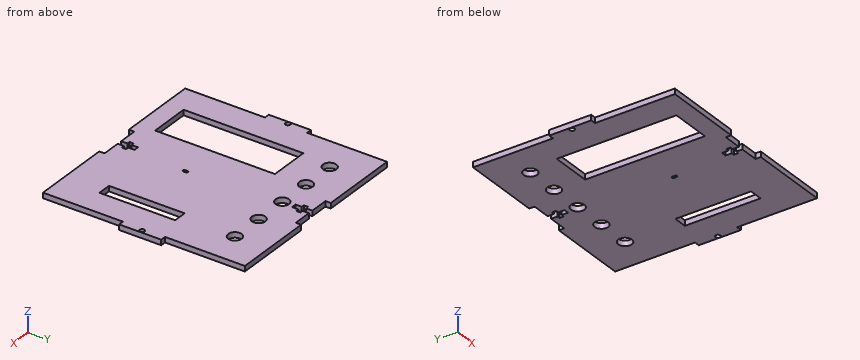
from build123d import *

# Parameters (mm, degrees)
SKETCH1_R           = 1.47
BOSS_EXTRUDE1_DEPTH = 1.5875
SKETCH3_W           = 8
SKETCH3_H           = 45
CUT_EXTRUDE1_DEPTH  = 88.184638842
SKETCH4_W           = 24
SKETCH4_H           = 71.2
CUT_EXTRUDE2_DEPTH  = 88.184638842
CUT_EXTRUDE4_DEPTH  = 88.184638842
SKETCH6_R           = 4
CUT_EXTRUDE5_DEPTH  = 88.184638842


with BuildPart() as part:
    # Sketch1 → Boss-Extrude1 (new, symmetric)
    with BuildSketch(Plane.XY):
        Polygon((-12.5, 60), (-60, 60), (-60, 12.5), (-63.175, 12.5), (-63.175, -12.5), (-60, -12.5), (-60, -60), (-12.5, -60), (-12.5, -56.825), (-1.47, -56.825), (-1.47, -53.125), (-3.25, -53.125), (-3.25, -50.525), (-1.47, -50.525), (-1.47, -46.825), (1.47, -46.825), (1.47, -50.525), (3.25, -50.525), (3.25, -53.125), (1.47, -53.125), (1.47, -56.825), (12.5, -56.825), (12.5, -60), (60, -60), (60, -12.5), (63.175, -12.5), (63.175, 12.5), (60, 12.5), (60, 60), (12.5, 60), (12.5, 56.825), (1.47, 56.825), (1.47, 53.125), (3.25, 53.125), (3.25, 50.525), (1.47, 50.525), (1.47, 46.825), (-1.47, 46.825), (-1.47, 50.525), (-3.25, 50.525), (-3.25, 53.125), (-1.47, 53.125), (-1.47, 56.825), (-12.5, 56.825), align=None)
        with Locations((-61.5875, 0)):
            Circle(SKETCH1_R, mode=Mode.SUBTRACT)
        with Locations(Location((61.5875, 0, 0), (0, 0, 180))):
            Circle(SKETCH1_R, mode=Mode.SUBTRACT)
    extrude(amount=BOSS_EXTRUDE1_DEPTH, both=True)

    # Sketch3 → Cut-Extrude1 (cut, through all)
    with BuildSketch(Plane(origin=(0, 0, -1.5875), x_dir=(-1, 0, 0), z_dir=(0, 0, -1))):
        with Locations((-40.3, -15)):
            Rectangle(SKETCH3_W, SKETCH3_H)
    extrude(amount=-CUT_EXTRUDE1_DEPTH, mode=Mode.SUBTRACT)

    # Sketch4 → Cut-Extrude2 (cut, through all)
    with BuildSketch(Plane(origin=(0, 0, -1.5875), x_dir=(-1, 0, 0), z_dir=(0, 0, -1))):
        with Locations((31.2, -13.494459363)):
            Rectangle(SKETCH4_W, SKETCH4_H)
    extrude(amount=-CUT_EXTRUDE2_DEPTH, mode=Mode.SUBTRACT)

    # Sketch5 → Cut-Extrude4 (cut, through all)
    with BuildSketch(Plane(origin=(0, 0, -1.5875), x_dir=(-1, 0, 0), z_dir=(0, 0, -1))):
        with BuildLine():
            Line((-3.324117887, -16.45), (-3.949848491, -16.45))
            ThreePointArc((-3.949848491, -16.45), (-4.214195834, -16.350200736), (-4.346634826, -16.10060241))
            ThreePointArc((-4.346634826, -16.10060241), (-4.416532026, -15), (-4.346634826, -13.89939759))
            ThreePointArc((-4.346634826, -13.89939759), (-4.214195834, -13.649799264), (-3.949848491, -13.55))
            Line((-3.949848491, -13.55), (-3.324117887, -13.55))
            ThreePointArc((-3.324117887, -13.55), (-3.041275174, -13.667157288), (-2.924117887, -13.95))
            Line((-2.924117887, -13.95), (-2.924117887, -16.05))
            ThreePointArc((-2.924117887, -16.05), (-3.041275174, -16.332842712), (-3.324117887, -16.45))
        make_face()
    extrude(amount=-CUT_EXTRUDE4_DEPTH, mode=Mode.SUBTRACT)

    # Sketch6 → Cut-Extrude5 (cut, through all)
    with BuildSketch(Plane(origin=(0, 0, -1.5875), x_dir=(-1, 0, 0), z_dir=(0, 0, -1))):
        with Locations((40, 40)):
            Circle(SKETCH6_R)
        with Locations((20, 40)):
            Circle(SKETCH6_R)
        with Locations((0, 40)):
            Circle(SKETCH6_R)
        with Locations((-20, 40)):
            Circle(SKETCH6_R)
        with Locations((-40, 40)):
            Circle(SKETCH6_R)
    extrude(amount=-CUT_EXTRUDE5_DEPTH, mode=Mode.SUBTRACT)


solid = part.part
CAD build for the part. Positions are in the model's coordinates, mm. Round coordinates to 2 decimals unless told otherwise and drop trailing zeros. Order: outer loops, then holes, each group sorted by start corner. A loop starts at its lowest first (then second) coordinate and runs counter-clockwise, first axis right, second up. Notation, with made-up numbers: (-26, 62) -> (23, 62) arc R22 cw to (23, 81) -> close; hole circle Ø4 at (-2.5, -22). An arc over 180 degrees is marked (long way). Write item = value, one per line. Start each with the question number.
(1) Cut at A-A, the plane y = -39. List the corners of the cut face in (x, z).
(2) Cut at B-B, the plane x = 0. List the corners of the cut face in (y, z) (1 decimal), then the cut area to 3 significant figures.
(3) Pin check, flat tips, straight feed: P1, Ø0.9, axis at x = 2, z = 0.5, coming from the +Y side (3 decimals); P2, Ø1.6, axis at y = -48.5, z = 0.5, coming from the +X side; P3, Ø1.5, axis at y = -23.5, z = 1, coming from the -X side; P4, Ø1.5, axis at x = 43.5, y = -3, coming from the +Z side. Stop position of each tip, or through.
(4) Cut at D-D, the plane x = -40. List the corners of the cut face in (y, z).
(5) Probe line 1 (Y direction, x = -20.5, z = -0.7); line 2 (X direction, y = -7, z = 0.3) (3 decimals); line 3 (X direction, y = -31.5, z = 0.7). List the from-to ranges inside material, lowest first. Write a range as [from, to].
(6) Cut at C-C, the plane y = 40. List the corners of the cut face in (x, z).
Model answer:
q1.outline = (-60, -1.59) -> (-43.2, -1.59) -> (-43.2, 1.59) -> (-60, 1.59) -> close; (-19.2, -1.59) -> (60, -1.59) -> (60, 1.59) -> (-19.2, 1.59) -> close
q2.outline = (-46.8, -1.6) -> (36, -1.6) -> (36, 1.6) -> (-46.8, 1.6) -> close; (44, -1.6) -> (46.8, -1.6) -> (46.8, 1.6) -> (44, 1.6) -> close
q2.area = 272 mm2
q3.P1 = 56.825
q3.P2 = 60
q3.P3 = -60
q3.P4 = through
q4.outline = (-60, -1.59) -> (-49.09, -1.59) -> (-49.09, 1.59) -> (-60, 1.59) -> close; (22.11, -1.59) -> (36, -1.59) -> (36, 1.59) -> (22.11, 1.59) -> close; (44, -1.59) -> (60, -1.59) -> (60, 1.59) -> (44, 1.59) -> close
q5.line_1 = [-60, -49.09], [22.11, 36.03], [43.97, 60]
q5.line_2 = [-63.175, -43.2], [-19.2, 36.3], [44.3, 63.175]
q5.line_3 = [-60, -43.2], [-19.2, 36.3], [44.3, 60]
q6.outline = (-60, -1.59) -> (-44, -1.59) -> (-44, 1.59) -> (-60, 1.59) -> close; (-36, -1.59) -> (-24, -1.59) -> (-24, 1.59) -> (-36, 1.59) -> close; (-16, -1.59) -> (-4, -1.59) -> (-4, 1.59) -> (-16, 1.59) -> close; (4, -1.59) -> (16, -1.59) -> (16, 1.59) -> (4, 1.59) -> close; (24, -1.59) -> (36, -1.59) -> (36, 1.59) -> (24, 1.59) -> close; (44, -1.59) -> (60, -1.59) -> (60, 1.59) -> (44, 1.59) -> close
